Check sheet for the modelled part. Datum: model origin and axes. Units: mm. Face numbers are marked on the shaded views. A direction names the side the tool comes from. Coordinates: 2 decimals unless noted, no trailing zeros. Loops run counter-clockwise (first coordinate to the right, second up) from the corner with the lowest first, then second, coordinate; pieces in that order, holes last. Notation, with made-up numbers: (55, 83.5) - (80, 83.5) arc R23 cw to (80, 91.5) - close; hole circle Ø5 at (22, 60). An arc over 180 degrees is marked (long way). Use a Markdown table: item, result. Add a question column.
1) Sectioned sample at B-B, the plane z = 51. Enter the section's corners in (x, y), then the cut area to 3 significant figures.
2) Go/stop test with flat-tipped pins: P1, Ø3, axis at x = -22, y = 4, coming from the +Z side; P2, Ø12, axis at y = 25.5, z = 86.5, coming from the -X side. Record where each tip stops, or that it passes through.
3) Sectioned sample at D-D, the plane x = -60. Enter the section's corners in (y, z).
4) Sectioned sample at C-C, the plane y = 34. Enter the section's corners in (x, z).
5) Tool access check on the marked faces 4, 5 and 6. Record the directions out of +Z, -Z, +X, -X, +Y, -Y that give a thin tool (end or side, any length) a straight path to the whole face; none if there is none.
6) Draft check along Y on the marked faces 1, 2 and 3. Enter one of: pulls with the +Y half, pulls with the -Y half, needs draft (parallel to the pull), parting line crosses it, or undercut.
7) Thickness scan on line 1 (Y direction, x = -32, z = 69.5); line 2 (Z direction, x = -54.5, y = 8); line 3 (X direction, y = 50, z = 63.5). Record the ranges inside material, lowest first.
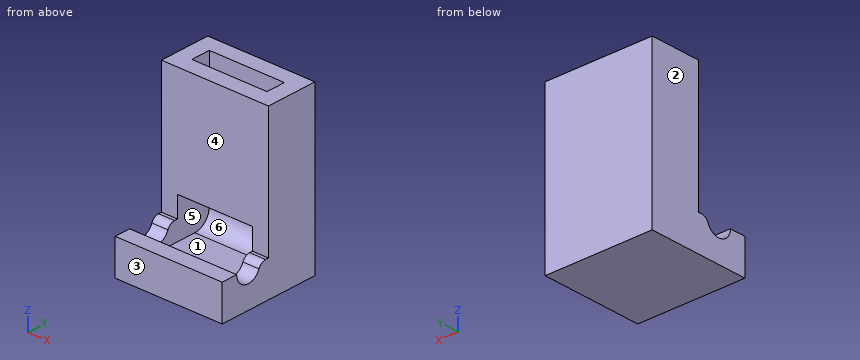
from build123d import *

# Parameters (mm, degrees)
F1_DEPTH  = 67
F2_W      = 47
F2_H      = 12
F3_DEPTH  = 92
F4_DEPTH  = 92
F5_W      = 47
F5_H      = 22
F6_DEPTH  = 12
F8_DEPTH  = 22
F9_R      = 9.99999
F11_DEPTH = 83
F12_R     = 5


# Not quite as in the source:
# - a fillet or chamfer is up to 0.001 mm smaller than in the source, because OpenCascade refuses the exact size


with BuildPart() as f1:
    # F0 (on Right) → F1 (new body)
    with BuildSketch(Plane.YZ):
        Polygon((0, 22), (0, 0), (64, 0), (64, 22), (64, 102), (32, 102), (32, 22), align=None)
    extrude(amount=-F1_DEPTH)

    # F2 (on face) → F3 (join)
    with BuildSketch(Plane.XY.offset(102)):
        with Locations((-33.5, 48)):
            Rectangle(F2_W, F2_H)
    extrude(amount=-F3_DEPTH)

    # F2 (on face) → F4 (cut)
    with BuildSketch(Plane.XY.offset(102)):
        with Locations((-33.5, 48)):
            Rectangle(F2_W, F2_H)
    extrude(amount=-F4_DEPTH, mode=Mode.SUBTRACT)

    # F5 (on face) → F6 (cut)
    with BuildSketch(Plane.XY.offset(22)):
        with Locations((-33.5, 21)):
            Rectangle(F5_W, F5_H)
    extrude(amount=-F6_DEPTH, mode=Mode.SUBTRACT)

    # F7 (on face) → F8 (cut)
    with BuildSketch(Plane.XZ.offset(-32)):
        Polygon((-57, 22), (-57, 10), (-10, 10), (-10, 22), (-10, 35), (-57, 35), align=None)
    extrude(amount=-F8_DEPTH, mode=Mode.SUBTRACT)

    # F9 (radius 10 in the source; OpenCascade refuses exactly that, so slightly less here)
    f9_edges = [f1.edges().sort_by_distance(p)[0] for p in [
        (-33.5, 54, 10),
        (-33.5, 42, 35),
    ]]
    fillet(f9_edges, radius=F9_R)

    # F10 (on face) → F11 (cut)
    with BuildSketch(Plane.YZ):
        with BuildLine():
            ThreePointArc((10, 22), (18, 14), (26, 22))
            Line((26, 22), (10, 22))
        make_face()
    extrude(amount=-F11_DEPTH, mode=Mode.SUBTRACT)

    # F12
    f12_edges = [f1.edges().sort_by_distance(p)[0] for p in [
        (-5, 26, 22),
        (-62, 26, 22),
    ]]
    fillet(f12_edges, radius=F12_R)


solid = f1.part
Solved:
| question | item | result |
|---|---|---|
| 1 | outline | (-67, 32) - (0, 32) - (0, 64) - (-67, 64) - close; hole (-57, 42) - (-10, 42) - (-10, 54) - (-57, 54) - close |
| 1 | area | 1,580 mm2 |
| 2 | P1 | stops at z = 22 |
| 2 | P2 | passes through |
| 3 | outline | (0, 0) - (64, 0) - (64, 102) - (32, 102) - (32, 22) - (30, 22) arc R5 ccw to (25.38, 18.92) arc R8 cw to (10, 22) - (0, 22) - close |
| 4 | outline | (-67, 0) - (0, 0) - (0, 102) - (-67, 102) - close; hole (-57, 10) - (-10, 10) - (-10, 35.2) - (-57, 35.2) - close |
| 5 | face 4 | +Z, +X, -X, -Y |
| 5 | face 5 | none |
| 5 | face 6 | +Z |
| 6 | face 1 | undercut |
| 6 | face 2 | needs draft |
| 6 | face 3 | pulls with the -Y half |
| 7 | line 1 | y = 32 to 42, 54 to 64 |
| 7 | line 2 | z = 0 to 22 |
| 7 | line 3 | x = -67 to -57, -10 to 0 |
